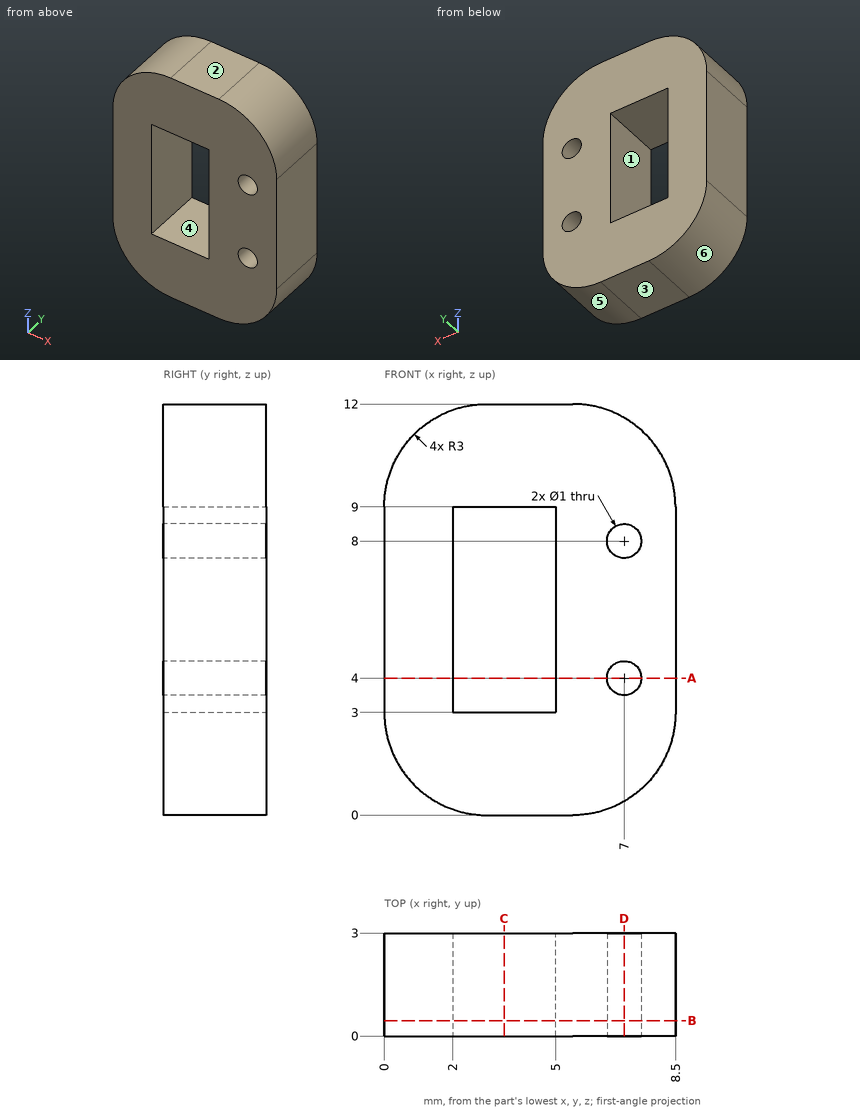
Verification items for this drawing (mm, ordinates from the low corner). A direction names the side the tool comes from. Give positions to 0.01 mm unless a question says otherwise; leave off trailing zeros. Loops run counter-clockwise (first coordinate to the right, second up) from the corner with the lowest first, then second, coordinate; pieces in that order, holes last. Notation, with made-up numbers: M 20.25,79.25 L 57.25,79.25 A29 cw 57.25,116.25 Z; hole C -26,52 d3. An arc over 180 degrees is marked long. Answer as a JSON object with one key per item and string values. Group by question number.
Item 1: Sectioned sample at A-A on z = 4. Record the boundary of the cut face in (x, y), plus the area to 3 significant figures.
Item 2: Access from +Z, -Z, +X, -X, +Y, -Y to the whole of each face (thin tool, end or side, straight path). Record for the marked faces 1 and 2.
Item 3: Sectioned sample at B-B on y = 0.45. Record the boundary of the cut face in (x, z).
Item 4: Sectioned sample at C-C on x = 3.5. Record the boundary of the cut face in (y, z).
Item 5: Mould release check, pull along X, two halves, no side actions. Record for the marked faces 3, 4, 5 and 6: pulls with the +X half, pulls with the -X half, needs draft (parallel to the pull), parting line crosses it, or undercut.
Item 6: Sectioned sample at D-D on x = 7. Record the boundary of the cut face in (y, z).
Item 7: Material ranges on L1, parallel to X at y = 1.9, z = 4; L2, parallel to Z at x = 7, y = 1.9; L3, parallel to Z at x = 4.75, y = 1.55, recorded low to high.
Findings below:
{
 "1": {"outline": "M 0,0 L 2,0 L 2,3 L 0,3 Z; M 5,0 L 6.5,0 L 6.5,3 L 5,3 Z; M 7.5,0 L 8.5,0 L 8.5,3 L 7.5,3 Z", "area": "13.5 mm2"},
 "2": {"face 1": "+Y, -Y", "face 2": "+Z, +X, -X, +Y, -Y"},
 "3": {"outline": "M 0,3 A3 ccw 3,0 L 5.5,0 A3 ccw 8.5,3 L 8.5,9 A3 ccw 5.5,12 L 3,12 A3 ccw 0,9 Z; hole M 2,3 L 5,3 L 5,9 L 2,9 Z; hole C 7,4 d1; hole C 7,8 d1"},
 "4": {"outline": "M 0,0 L 3,0 L 3,3 L 0,3 Z; M 0,9 L 3,9 L 3,12 L 0,12 Z"},
 "5": {"face 3": "needs draft", "face 4": "undercut", "face 5": "pulls with the +X half", "face 6": "pulls with the -X half"},
 "6": {"outline": "M 0,0.4 L 3,0.4 L 3,3.5 L 0,3.5 Z; M 0,4.5 L 3,4.5 L 3,7.5 L 0,7.5 Z; M 0,8.5 L 3,8.5 L 3,11.6 L 0,11.6 Z"},
 "7": {"L1": "0 to 2, 5 to 6.5, 7.5 to 8.5", "L2": "0.4 to 3.5, 4.5 to 7.5, 8.5 to 11.6", "L3": "0 to 3, 9 to 12"}
}
